Work out the finished part from the listing and answer in its coordinate system (mm). Face numbers are marked on the shaded views. Coordinates: 2 decimals unless noted, no trailing zeros. Write each loop counter-clockwise with the first axis right and the second up, starting at its lowest first coordinate (ties: lowest second). Pieces come first, ordered by that corner, then holes. Notation, with made-up numbers: (8, 71) - (56, 71) arc R28 ccw to (56, 95) - close; hole circle Ø9 at (-37, 42). An arc over 180 degrees is marked (long way). Use CSV: the item, a comma, the result in double quotes. Start each with the question number.
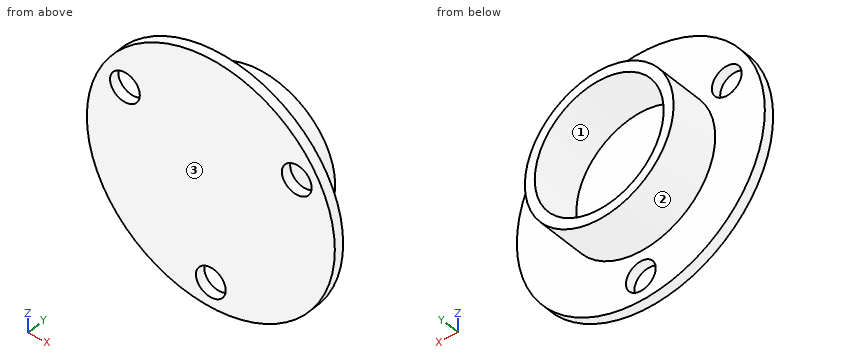
from build123d import *

# Parameters (mm, degrees)
SKETCH2_R           = 12.5
SKETCH2_R_2         = 1.5
BOSS_EXTRUDE1_DEPTH = 1
SKETCH3_R           = 7.5
SKETCH3_R_2         = 6.5
BOSS_EXTRUDE2_DEPTH = 5


with BuildPart() as part:
    # Sketch2 → Boss-Extrude1 (new body)
    with BuildSketch(Plane(origin=(0, 0, 0), x_dir=(1, 0, 0), z_dir=(0, 1, 0))):
        Circle(SKETCH2_R)
        with Locations((0, 10)):
            Circle(SKETCH2_R_2, mode=Mode.SUBTRACT)
        with Locations((8.660254038, -5)):
            Circle(SKETCH2_R_2, mode=Mode.SUBTRACT)
        with Locations((-8.660254038, -5)):
            Circle(SKETCH2_R_2, mode=Mode.SUBTRACT)
    extrude(amount=BOSS_EXTRUDE1_DEPTH)

    # Sketch3 → Boss-Extrude2 (add)
    with BuildSketch(Plane(origin=(0, 1, 0), x_dir=(1, 0, 0), z_dir=(0, 1, 0))):
        Circle(SKETCH3_R)
        Circle(SKETCH3_R_2, mode=Mode.SUBTRACT)
    extrude(amount=BOSS_EXTRUDE2_DEPTH)


solid = part.part
Item 1: A cutting plane is placed at A-A (z = 5). Determine the outline of the cut face in (x, y).
Item 2: A cutting plane is placed at C-C (z = 0). Determine the outline of the cut face in (x, y), then the cut area to 3 significant figures.
Item 3: Each of these flat-tipped pins is pushed along its axis until it touches: pin 1 (1.5 mm diameter, centred on y = 1, z = -8, fed in from +X); pin 2 (3.5 mm diameter, centred on x = 8.66, z = 5, fed in from +Y); pin 3 (2 mm diameter, centred on y = 1, z = -9.5, fed in from -X). Where does it stop, or does it pass through?
Item 4: Straight lines are drawn through the part: probe 1 along X at (y, z) = (0.45, -10); probe 2 along X at (y, z) = (0.6, 5); probe 3 along Z at (x, y) = (0, 2.25). For each, find the intervals that lie inside material, in ascending order. Write a range as [from, to].
Item 5: Determine the mould class of the marked faces 1, 2 and 3 for opening direction Z: +Z half, -Z half, draft (parallel to the pull), parting line (faces both ways), or undercut.
Item 6: A cutting plane is placed at D-D (x = -3.5). Determine the outline of the cut face in (y, z), then the cut area to 3 significant figures.
Item 7: A cutting plane is placed at B-B (x = 0). Determine the outline of the cut face in (y, z).
Calculated:
1,outline,"(-11.46, 0) - (-10.16, 0) - (-10.16, 1) - (-11.46, 1) - close; (-7.16, 0) - (7.16, 0) - (7.16, 1) - (5.59, 1) - (5.59, 6) - (4.15, 6) - (4.15, 1) - (-4.15, 1) - (-4.15, 6) - (-5.59, 6) - (-5.59, 1) - (-7.16, 1) - close; (10.16, 0) - (11.46, 0) - (11.46, 1) - (10.16, 1) - close"
2,outline,"(-12.5, 0) - (12.5, 0) - (12.5, 1) - (7.5, 1) - (7.5, 6) - (6.5, 6) - (6.5, 1) - (-6.5, 1) - (-6.5, 6) - (-7.5, 6) - (-7.5, 1) - (-12.5, 1) - close"
2,area,"35.0 mm²"
3,pin 1,"stops at x = 10.18"
3,pin 2,"stops at y = 1"
3,pin 3,"stops at x = -9.17"
4,probe 1,"x = [-7.5, -1.5], [1.5, 7.5]"
4,probe 2,"x = [-11.46, -10.16], [-7.16, 7.16], [10.16, 11.46]"
4,probe 3,"z = [-7.5, -6.5], [6.5, 7.5]"
5,face 1,"undercut"
5,face 2,"parting line"
5,face 3,"draft"
6,outline,"(0, -12) - (1, -12) - (1, -6.63) - (6, -6.63) - (6, -5.48) - (1, -5.48) - (1, 5.48) - (6, 5.48) - (6, 6.63) - (1, 6.63) - (1, 12) - (0, 12) - close"
6,area,"35.6 mm²"
7,outline,"(0, -12.5) - (1, -12.5) - (1, -11.5) - (0, -11.5) - close; (0, -8.5) - (1, -8.5) - (1, -7.5) - (6, -7.5) - (6, -6.5) - (1, -6.5) - (1, 6.5) - (6, 6.5) - (6, 7.5) - (1, 7.5) - (1, 12.5) - (0, 12.5) - close"
